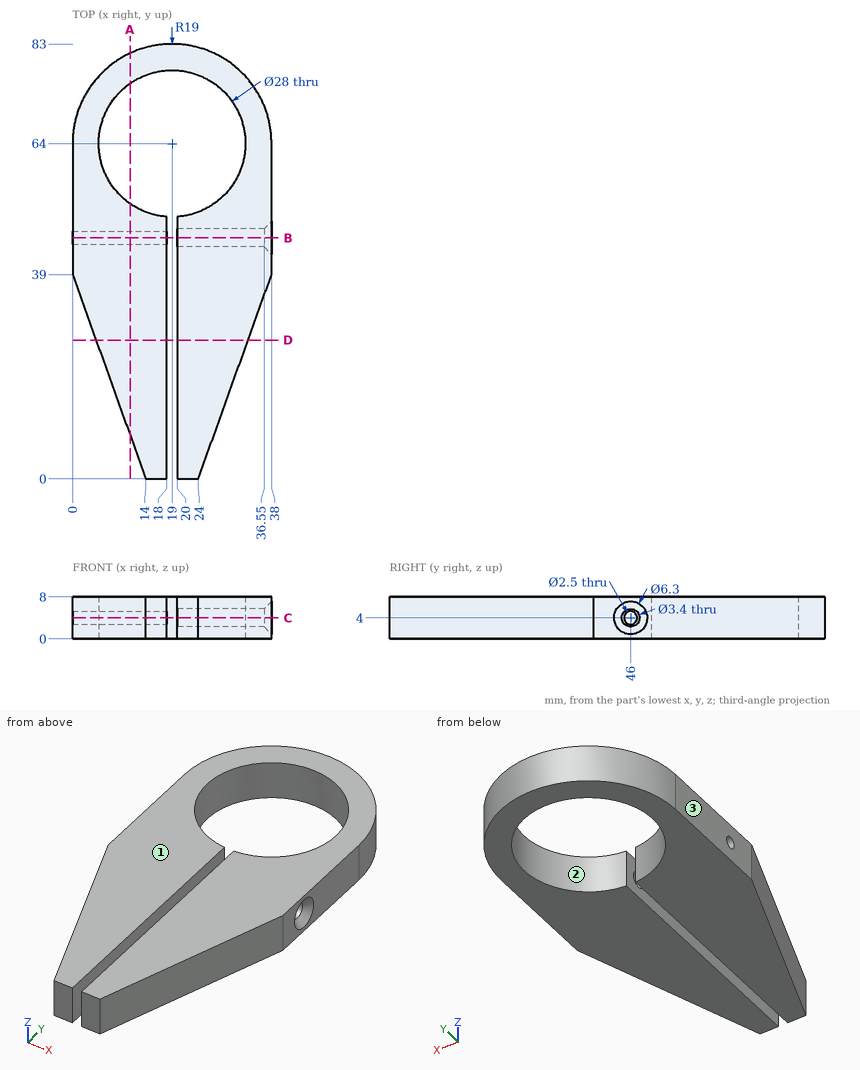
Print and shaded views of the part. All mm, measured from the part's lowest x, y and z. Coordinates: 2 decimals unless noted, no trailing zeros. Order: outer loops, then holes, each group sorted by start corner. A loop starts at its lowest first (then second) coordinate and runs counter-clockwise, first axis right, second up. Notation, with made-up numbers: M -24,88 L 32,88 A20 ccw 32,105 Z; hole C 67,-1.5 d7. An arc over 180 degrees is marked long. Answer as CSV lines item,"result".
1) Flat gauge pins, fed straight in: P1, Ø3, axis at y = 72, z = 4, coming from the -X side; P2, Ø4, axis at y = 25.5, z = 2, coming from the -X side. Where does each tip first touch, or does it go through?
Verdict:
P1,"x = 1.15"
P2,"x = 4.13"
2) Mould opens along X. For the marked faces 1, 2 and 3 say: released by +X, released by -X, zero draft, split by the parting line, or undercut.
Verdict:
face 1,"zero draft"
face 2,"undercut"
face 3,"released by -X"
3) Cut at D-D (y = 26.5). List the corners of the cut face in (x, z).
Verdict:
outline,"M 4.49,0 L 18,0 L 18,8 L 4.49,8 Z; M 20,0 L 33.51,0 L 33.51,8 L 20,8 Z"
4) Cut at A-A (x = 11). List the corners of the cut face in (y, z), then the cut area to 3 significant figures.
Verdict:
outline,"M 8.36,0 L 52.51,0 L 52.51,8 L 8.36,8 Z; M 75.49,0 L 81.23,0 L 81.23,8 L 75.49,8 Z; hole C 46,4 d2.5"
area,"394 mm2"
5) Cut at C-C (z = 4). List the corners of the cut face in (x, y), then the cut area to 3 significant figures.
Verdict:
outline,"M 0,39 L 14,0 L 18,0 L 18,44.75 L 0,44.75 Z; M 0,47.25 L 18,47.25 L 18,50.04 A14 cw long 20,50.04 L 20,47.7 L 36.55,47.7 L 38,49.15 L 38,64 A19 ccw 0,64 Z; M 20,0 L 24,0 L 38,39 L 38,42.85 L 36.55,44.3 L 20,44.3 Z"
area,"1,630 mm2"
6) Drill centre lines: L1, parallel to Z at x = 10.75, y = 46; L2, parallel to X at y = 64, z = 2.5; L3, parallel to Y at x = 22, z = 5.5. Where is each one in solid material? Low to high. Write a range as from..to.
Verdict:
L1,"0..2.75, 5.25..8"
L2,"0..5, 33..38"
L3,"0..45.2, 46.8..50.33, 77.67..82.76"
7) Cut at B-B (y = 46). List the corners of the cut face in (x, z), then the cut area to 3 significant figures.
Verdict:
outline,"M 0,0 L 18,0 L 18,2.75 L 0,2.75 Z; M 0,5.25 L 18,5.25 L 18,8 L 0,8 Z; M 20,0 L 38,0 L 38,0.85 L 36.55,2.3 L 20,2.3 Z; M 20,5.7 L 36.55,5.7 L 38,7.15 L 38,8 L 20,8 Z"
area,"180 mm2"
